Could you check a few things on this model? Use its own coordinates, in mm. A direction names the side the tool comes from. Give positions to 0.01 mm unless a question says otherwise; leave off trailing zeros. Loops run counter-clockwise (first coordinate to the right, second up) from the corner with the lowest first, then second, coordinate; pieces in that order, holes last.
1. For faces 4 (the flat face through (254, 51, 16)), 5 (the flat face through (69.908, 127.356, 15.653)), 6 (the cylindrical face through (113.338, 139.878, 15.726)), 7 (the flat face through (152, 127, 16)), which set-ups out of +Z, -Z, +X, -X, +Y, -Y let a thin tool reach every point of the face, with its end or its side?
2. Imagine slicing it at B-B (x = 176). List the corners of the cut face in (y, z) for me, plus the area to 3 significant figures.
3. Imagine slicing it at A-A (y = 50.5). List the corners of the cut face in (x, z) for me, plus the area to 3 significant figures.
4. Imagine slicing it at D-D (y = 63.5). List the corners of the cut face in (x, z) for me, plus the area to 3 significant figures.
5. Imagine slicing it at C-C (z = 9.5). List the corners of the cut face in (x, y) for me, plus the area to 3 significant figures.
6. For P1, Ø5, axis at y = 105, z = 14.5, coming from the +X side; P2, Ø5.5, axis at y = 38.1, z = 25.4, coming from the -X side; P3, Ø9.5, axis at x = 150.5, z = 16.5, coming from the +Y side; P4, Ø3, axis at x = 152, z = 14, coming from the +Y side, each with a flat end and sliding along its axis, tell me the tip position at first contact or that it passes through.
7. I need wall thicknesses on line 1 along Z through (x, y) = (42, 38); line 2 along X through (y, z) = (41.5, 19.5); line 3 along Y through (x, z) = (179.5, 28). Which ranges of each line are inside material? Lowest first, please.
8. Thinking about a two-plate mould opening in X: for faces 1 (the cylindrical face through (142.536, 143.239, 15.653)), 2 (the flat face through (266.7, 63, 16)), 3 (the cylindrical face through (44.36, 60.2, 24.67)), which applies, +X half, -X half, draft (parallel to the pull), parting line (faces both ways), or undercut?
```python
from build123d import *

# Parameters (mm, degrees)
BOSS_EXTRUDE1_DEPTH = 50.8
SKETCH3_R           = 3.3782
CUT_EXTRUDE1_DEPTH  = 25.4
SKETCH4_R           = 3.3782
CUT_EXTRUDE2_DEPTH  = 25.4
SKETCH7_W           = 279.740966103
SKETCH7_H           = 194.949015238
CUT_EXTRUDE5_DEPTH  = 19.05
SKETCH8_W           = 228.6
SKETCH8_H           = 25.4
CUT_EXTRUDE6_DEPTH  = 39.37
SKETCH9_R           = 3.3782
CUT_EXTRUDE7_DEPTH  = 27.94
CUT_EXTRUDE8_DEPTH  = 40.64
SKETCH12_W          = 1.27
SKETCH12_H          = 31.75
CUT_EXTRUDE9_DEPTH  = 16.51
CUT_EXTRUDE10_REACH = 33.75
SKETCH13_R          = 3.3782


with BuildPart() as part:
    # Sketch2 → Boss-Extrude1 (new body)
    with BuildSketch(Plane.XY):
        with BuildLine():
            Line((254, 0), (266.7, 0))
            Line((266.7, 0), (266.7, 101.6))
            Line((266.7, 101.6), (203.962, 152.4))
            Line((203.962, 152.4), (165.862, 152.4))
            ThreePointArc((165.862, 152.4), (152.4, 138.938), (138.938, 152.4))
            Line((138.938, 152.4), (100.838, 152.4))
            Line((100.838, 152.4), (38.1, 101.6))
            Line((38.1, 101.6), (38.1, 0))
            Line((38.1, 0), (50.8, 0))
            Line((50.8, 0), (50.8, 76.2))
            Line((50.8, 76.2), (254, 76.2))
            Line((254, 76.2), (254, 0))
        make_face()
    extrude(amount=BOSS_EXTRUDE1_DEPTH)

    # Sketch3 → Cut-Extrude1 (cut)
    with BuildSketch(Plane.ZY.offset(-38.1)):
        with Locations((25.4, 63.5)):
            Circle(SKETCH3_R)
        with Locations((25.4, 38.1)):
            Circle(SKETCH3_R)
    extrude(amount=-CUT_EXTRUDE1_DEPTH, mode=Mode.SUBTRACT)

    # Sketch4 → Cut-Extrude2 (cut)
    with BuildSketch(Plane(origin=(266.7, 0, 0), x_dir=(0, 0, -1), z_dir=(1, 0, 0))):
        with Locations((-25.4, 63.5)):
            Circle(SKETCH4_R)
        with Locations((-25.4, 38.1)):
            Circle(SKETCH4_R)
    extrude(amount=-CUT_EXTRUDE2_DEPTH, mode=Mode.SUBTRACT)

    # Sketch7 → Cut-Extrude5 (cut)
    with BuildSketch(Plane.XY.offset(50.8)):
        with Locations((152.037641236, 76.2)):
            Rectangle(SKETCH7_W, SKETCH7_H)
    extrude(amount=-CUT_EXTRUDE5_DEPTH, mode=Mode.SUBTRACT)

    # Sketch8 → Cut-Extrude6 (cut)
    with BuildSketch(Plane.XY.offset(31.75)):
        with Locations((152.4, 12.7)):
            Rectangle(SKETCH8_W, SKETCH8_H)
    extrude(amount=-CUT_EXTRUDE6_DEPTH, mode=Mode.SUBTRACT)

    # Sketch9 → Cut-Extrude7 (cut)
    with BuildSketch(Plane(origin=(0, 152.4, 0), x_dir=(1, 0, 0), z_dir=(0, 1, 0))):
        with Locations((116.713, -15.875)):
            Circle(SKETCH9_R)
        with Locations((188.087, -15.875)):
            Circle(SKETCH9_R)
    extrude(amount=-CUT_EXTRUDE7_DEPTH, mode=Mode.SUBTRACT)

    # Sketch10 → Cut-Extrude8 (cut)
    with BuildSketch(Plane.XY.offset(31.75)):
        Polygon((68.372272223, 101.6), (99.741272223, 127), (205.058727777, 127), (236.427727777, 101.6), align=None)
    extrude(amount=-CUT_EXTRUDE8_DEPTH, mode=Mode.SUBTRACT)

    # Sketch12 → Cut-Extrude9 (cut)
    with BuildSketch(Plane(origin=(0, 152.4, 0), x_dir=(1, 0, 0), z_dir=(0, 1, 0))):
        with Locations((153.035, -15.875)):
            Rectangle(SKETCH12_W, SKETCH12_H)
        with Locations((151.765, -15.875)):
            Rectangle(SKETCH12_W, SKETCH12_H)
    extrude(amount=-CUT_EXTRUDE9_DEPTH, mode=Mode.SUBTRACT)

    # Sketch13 → Cut-Extrude10 (cut, up to next)
    with BuildSketch(Plane.XY.offset(31.75), mode=Mode.PRIVATE) as cut_extrude10_sk1:
        with Locations((116.078, 95.25)):
            Circle(SKETCH13_R)
    cut_extrude10_tool1 = extrude(cut_extrude10_sk1.sketch, amount=-CUT_EXTRUDE10_REACH, mode=Mode.PRIVATE) & part.part
    add(cut_extrude10_tool1.solids().sort_by_distance((116.078, 95.25, 31.75))[0], mode=Mode.SUBTRACT)
    # Sketch13 → Cut-Extrude10 (cut, up to next)
    with BuildSketch(Plane.XY.offset(31.75), mode=Mode.PRIVATE) as cut_extrude10_sk2:
        with Locations((194.564, 95.25)):
            Circle(SKETCH13_R)
    cut_extrude10_tool2 = extrude(cut_extrude10_sk2.sketch, amount=-CUT_EXTRUDE10_REACH, mode=Mode.PRIVATE) & part.part
    add(cut_extrude10_tool2.solids().sort_by_distance((194.564, 95.25, 31.75))[0], mode=Mode.SUBTRACT)


solid = part.part
```
Derived:
1. face 4: +Z, -Z, -Y
1. face 5: +Z, -Z, -X, +Y
1. face 6: +Y
1. face 7: +Z, -Z
2. outline: (76.2, 0) - (101.6, 0) - (101.6, 31.75) - (76.2, 31.75) - close; (127, 0) - (152.4, 0) - (152.4, 31.75) - (127, 31.75) - close
2. area: 1,610 mm2
3. outline: (38.1, 0) - (50.8, 0) - (50.8, 31.75) - (38.1, 31.75) - close; (254, 0) - (266.7, 0) - (266.7, 31.75) - (254, 31.75) - close
3. area: 806 mm2
4. outline: (38.1, 0) - (50.8, 0) - (50.8, 22.02) - (38.1, 22.02) - close; (38.1, 28.78) - (50.8, 28.78) - (50.8, 31.75) - (38.1, 31.75) - close; (254, 0) - (266.7, 0) - (266.7, 22.02) - (254, 22.02) - close; (254, 28.78) - (266.7, 28.78) - (266.7, 31.75) - (254, 31.75) - close
4. area: 635 mm2
5. outline: (38.1, 25.4) - (50.8, 25.4) - (50.8, 76.2) - (254, 76.2) - (254, 25.4) - (266.7, 25.4) - (266.7, 101.6) - (203.96, 152.4) - (165.86, 152.4) arc R13.46 cw to (153.67, 139) - (153.67, 135.89) - (151.13, 135.89) - (151.13, 139) arc R13.46 cw to (138.94, 152.4) - (100.84, 152.4) - (38.1, 101.6) - close; hole (68.37, 101.6) - (236.43, 101.6) - (205.06, 127) - (99.74, 127) - close; hole circle Ø6.76 at (116.08, 95.25); hole circle Ø6.76 at (194.56, 95.25)
5. area: 11,700 mm2
6. P1: stops at x = 265.59
6. P2: passes through
6. P3: stops at y = 140.7
6. P4: stops at y = 139.07
7. line 1: z = 0 to 22.02, 28.78 to 31.75
7. line 2: x = 38.1 to 50.8, 254 to 266.7
7. line 3: y = 76.2 to 101.6, 127 to 152.4
8. face 1: undercut
8. face 2: +X half
8. face 3: draft
